The model under review builds one solid part; all positions refer to its coordinate system, in mm. Face numbers are marked on the shaded views. A direction names the side the tool comes from. Round coordinates to 2 decimals unless told otherwise and drop trailing zeros. Write each loop counter-clockwise with the first axis right and the second up, starting at its lowest first coordinate (ties: lowest second). Pieces come first, ordered by that corner, then holes. Notation, with made-up numbers: M 60,79.5 L 95,79.5 A15 ccw 95,101.5 Z; hole C -16.75,-30.5 d10. An arc over 180 degrees is marked long. Write item = value, one per line. Start each with the question number.
Item 1: Take a section at B-B, the plane z = -3. Give the boundary of the cut face in (x, y), plus the area to 3 significant figures.
Item 2: To check wall thickness, follow line 1 along Z through (x, y) = (1.5, 2.5); line 2 along Z through (x, y) = (3.75, 5.25); line 3 along Y through (x, z) = (-0.25, -3). State the ranges of each line that lie inside material, in increasing order.
Item 3: The part is to be moulded in two halves that separate along X. For the marked faces 3, 4 and 5, say which applies: +X half, -X half, draft (parallel to the pull), parting line (faces both ways), or undercut.
Item 4: For pin 1 Ø2 at (y, z) = (-2.5, -6) entering from -X; pin 2 Ø4 at (y, z) = (-1.5, -3) entering from -X; pin 3 Ø1.5 at (y, z) = (-2.5, -6) entering from +X, all flat-tipped, find the tip position at first contact; note any pin that passes through.
Item 5: Take a section at D-D, the plane z = -4.5. Give the boundary of the cut face in (x, y).
Item 6: Take a section at C-C, the plane y = 0. Give the boundary of the cut face in (x, z), plus the area to 3 significant figures.
Item 7: Take a section at A-A, the plane x = 0. Give the boundary of the cut face in (y, z).
Item 8: Tool access review of the marked faces 1 and 2: name each direction out of +Z, -Z, +X, -X, +Y, -Y from which nothing blocks a thin tool from reaching the whole face with its end or side.
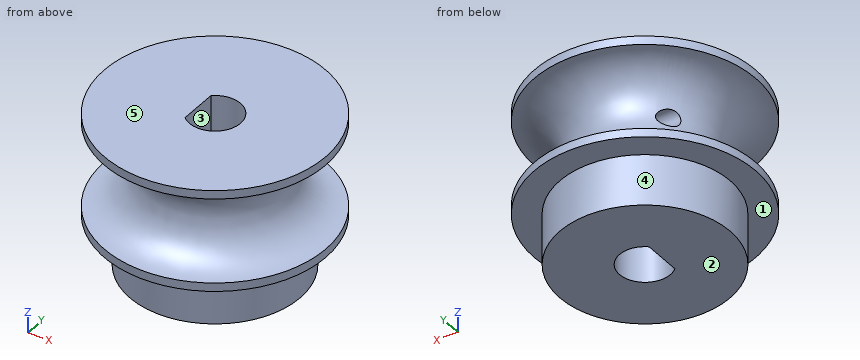
Autodesk Inventor part; units mm, degrees
ref_plane "작업 평면1" through (0, 0, -3) normal (0, 0, 1) x (1, 0, 0)
ref_plane "YZ Plane" through (0, 0, 0) normal (1, 0, 0) x (0, 1, 0)
ref_plane "XZ Plane" through (0, 0, 0) normal (0, 1, 0) x (-1, 0, 0)
sketch "스케치1" plane through (0, 0, 0) normal (1, 0, 0) x (0, 1, 0)
  line L0 (0, 0) -> (0, -9)
  line L1 (0, 0) -> (1.5, 0)
  line L2 (1.5, 0) -> (1.5, -9)
  line L3 (1.5, -9) -> (5, -9)
  line L4 (5, -9) -> (5, -6)
  line L5 (5, -6) -> (6.5, -6)
  line L6 (1.5, 0) -> (6.5, 0)
  line L7 (6.5, 0) -> (6.5, -0.5)
  line L8 (6.5, -3) -> (1.5, -3) construction
  line L9 (6.5, -6) -> (6.5, -5.5)
  arc A0 (6.5, -0.5) -> (6.5, -5.5) centre (6.5, -3) ccw
  dimension "d0" = 9
  dimension "d2" = 9
  dimension "d3" = 3
  dimension "d4" = 10
  dimension "d6" = 3
  dimension "d7" = 3
  dimension "d8" = 13
  dimension "d9" = 0.5
  dimension "d10" = 0.5
  dimension "d11" = 13
revolve "회전1" add sketch "스케치1" angle 360 about axis through (0, 0, 0) along (0, 0, -1)
sketch "스케치2" plane through (0, 0, -9) normal (0, 0, -1) x (-1, 0, 0)
  circle A0 centre (0, 0) radius 1.5
  line L0 (1, 1.118) -> (1, -1.118)
  dimension "d13" = 1
extrude "돌출1" add sketch "스케치2" against normal blind 9 contours A0 L0 picked at (1.1667, 0)
ref_plane "작업 평면1" through (0, 0, -3) normal (0, 0, 1) x (1, 0, 0)
sketch "스케치3" plane through (0, 0, -3) normal (0, 0, 1) x (1, 0, 0)
  line L0 (3.0429, 2.5) -> (-2.6844, 2.5)
  line L1 (-5.7069, 2.5) -> (4.2931, 2.5)
  line L2 (4.2931, 2.5) -> (4.2931, 3)
  line L3 (4.2931, 3) -> (-5.7069, 3)
  line L4 (-5.7069, 3) -> (-5.7069, 2.5)
  point P0 (0, 0)
  dimension "d16" = 0.5
  dimension "d17" = 2.5
  dimension "d18" = 10
revolve "회전2" cut sketch "스케치3" angle 360 about axis through (-5.7069, 2.5, -3) along (1, 0, 0)
properties part number "지름 핸들러"
Response values:
q1.outline = M -3.46,2 A4 ccw long 3.46,2 Z; M -2.65,3 L 2.65,3 A4 ccw Z; hole M -1,-1.12 A1.5 ccw long -1,1.12 Z
q1.area = 37.8 mm2
q2.line_1 = -9 to -3.5, -2.5 to 0
q2.line_2 = -6 to -5.5, -0.5 to 0
q2.line_3 = -3.99 to -1.48, 1.48 to 2, 3 to 3.99
q3.face_3 = undercut
q3.face_4 = parting line
q3.face_5 = draft
q4.pin_1 = -6.32
q4.pin_2 = -4.82
q4.pin_3 = 6.26
q5.outline = C 0,0 d9; hole M -1,-1.12 A1.5 ccw long -1,1.12 Z
q6.outline = M -6.5,-6 L -5,-6 L -5,-9 L -1,-9 L -1,0 L -6.5,0 L -6.5,-0.5 A2.5 cw -6.5,-5.5 Z; M 1.5,-9 L 5,-9 L 5,-6 L 6.5,-6 L 6.5,-5.5 A2.5 cw 6.5,-0.5 L 6.5,0 L 1.5,0 Z
q6.area = 65.9 mm2
q7.outline = M -6.5,-6 L -5,-6 L -5,-9 L -1.5,-9 L -1.5,0 L -6.5,0 L -6.5,-0.5 A2.5 cw -6.5,-5.5 Z; M 1.5,-9 L 5,-9 L 5,-6 L 6.5,-6 L 6.5,-5.5 A2.5 cw 6.5,-0.5 L 6.5,0 L 1.5,0 Z; hole C 2.5,-3 d1
q8.face_1 = -Z
q8.face_2 = -Z, +X, -X, +Y, -Y
